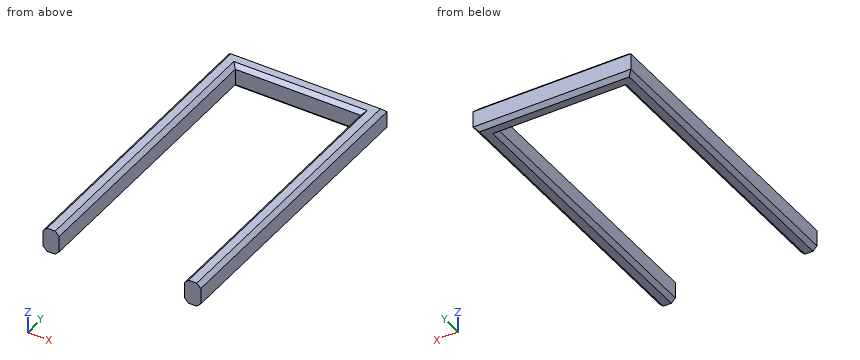
```python
from build123d import *

# Parameters (mm, degrees)
SKETCH1_W             = 8
SKETCH1_H             = 12
BOSS_EXTRUDE1_DEPTH   = 140
BOSS_EXTRUDE1_2_DEPTH = 140
SKETCH2_W             = 78
SKETCH2_H             = 12
BOSS_EXTRUDE2_DEPTH   = 8
CHAMFER1_SIZE         = 2


with BuildPart() as part:
    # Sketch1 → Boss-Extrude1 (new body)
    with BuildSketch(Plane(origin=(0, 0, 0), x_dir=(1, 0, 0), z_dir=(0, 1, 0))):
        with Locations((-35, 0)):
            Rectangle(SKETCH1_W, SKETCH1_H)
    extrude(amount=BOSS_EXTRUDE1_DEPTH)



with BuildPart() as body_2:
    # Sketch1 → Boss-Extrude1 2 (new body)
    with BuildSketch(Plane(origin=(0, 0, 0), x_dir=(1, 0, 0), z_dir=(0, 1, 0))):
        with Locations((35, 0)):
            Rectangle(SKETCH1_W, SKETCH1_H)
    extrude(amount=BOSS_EXTRUDE1_2_DEPTH)


with BuildPart() as part_1:
    add(part.part)

    add(body_2.part)  # Boss-Extrude2 merges body 2
    # Sketch2 → Boss-Extrude2 (add)
    with BuildSketch(Plane(origin=(0, 140, 0), x_dir=(1, 0, 0), z_dir=(0, 1, 0))):
        Rectangle(SKETCH2_W, SKETCH2_H)
    extrude(amount=BOSS_EXTRUDE2_DEPTH)

    # Chamfer1
    chamfer1_edges = [part_1.edges().sort_by_distance(p)[0] for p in [
        (0, 140, 6),
        (39, 74, 6),
        (39, 74, -6),
        (0, 148, 6),
        (0, 148, -6),
        (0, 140, -6),
        (31, 70, -6),
        (31, 70, 6),
        (-31, 70, 6),
        (-39, 74, 6),
        (-39, 74, -6),
        (-31, 70, -6),
    ]]
    chamfer(chamfer1_edges, length=CHAMFER1_SIZE)


solid = part_1.part
```
Build history of the part. All positions in model axes, mm. Give positions to 0.01 mm unless a question says otherwise; leave off trailing zeros. Loops run counter-clockwise (first coordinate to the right, second up) from the corner with the lowest first, then second, coordinate; pieces in that order, holes last. Notation, with made-up numbers: (-19, 71) -> (23, 71) arc R28 cw to (23, 97) -> close; hole circle Ø11 at (35.5, 67.25). An arc over 180 degrees is marked (long way). One line per question, with ' | ' between items. Start each with the question number.
1) Cut at B-B (x = -29). Give the cut face in (y, z).
2) Cut at A-A (y = 17.5). Give the cut face in (x, z).
3) Pin check, flat tip, straight feed: pin 1 (2.5 mm diameter, centred on x = -12, z = 2, fed in from -Y). Stop position of the tip, or through.
4) Cut at C-C (z = -2.25). Give the cut face in (x, y), plus the area to 3 significant figures.
5) Probe L1, parallel to X at y = 30, z = -2.25; L2, parallel to Y at x = -13, z = 1.5; L3, parallel to X at y = 31, z = 4.75. List the from-to ranges inside material, lowest first.
Return value:
1) outline: (140, -4) -> (142, -6) -> (146, -6) -> (148, -4) -> (148, 4) -> (146, 6) -> (142, 6) -> (140, 4) -> close
2) outline: (-39, -4) -> (-37, -6) -> (-33, -6) -> (-31, -4) -> (-31, 4) -> (-33, 6) -> (-37, 6) -> (-39, 4) -> close; (31, -4) -> (33, -6) -> (37, -6) -> (39, -4) -> (39, 4) -> (37, 6) -> (33, 6) -> (31, 4) -> close
3) pin 1: y = 140
4) outline: (-39, 0) -> (-31, 0) -> (-31, 140) -> (31, 140) -> (31, 0) -> (39, 0) -> (39, 148) -> (-39, 148) -> close | area: 2,860 mm^2
5) L1: -39 to -31, 31 to 39 | L2: 140 to 148 | L3: -38.25 to -31.75, 31.75 to 38.25
